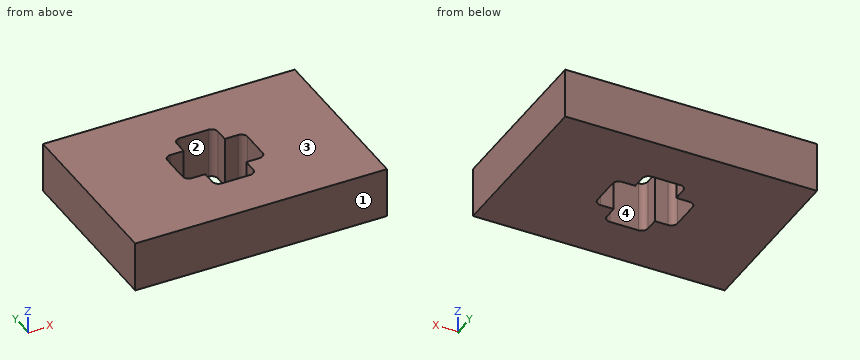
from build123d import *

# Parameters (mm, degrees)
SKETCH1_W           = 100
SKETCH1_H           = 70
BOSS_EXTRUDE1_DEPTH = 20


with BuildPart() as part:
    # Sketch1 → Boss-Extrude1 (new body)
    with BuildSketch(Plane.XY):
        Rectangle(SKETCH1_W, SKETCH1_H)
        with BuildLine():
            Line((-8.15, 13.4), (-8.15, 8.15))
            Line((-8.15, 8.15), (-13.4, 8.15))
            ThreePointArc((-13.4, 8.15), (-15.167766953, 7.417766953), (-15.9, 5.65))
            Line((-15.9, 5.65), (-15.9, -5.65))
            ThreePointArc((-15.9, -5.65), (-15.167766953, -7.417766953), (-13.4, -8.15))
            Line((-13.4, -8.15), (-8.15, -8.15))
            Line((-8.15, -8.15), (-8.15, -13.4))
            ThreePointArc((-8.15, -13.4), (-7.417766953, -15.167766953), (-5.65, -15.9))
            Line((-5.65, -15.9), (5.65, -15.9))
            ThreePointArc((5.65, -15.9), (7.417766953, -15.167766953), (8.15, -13.4))
            Line((8.15, -13.4), (8.15, -8.15))
            Line((8.15, -8.15), (13.4, -8.15))
            ThreePointArc((13.4, -8.15), (15.167766953, -7.417766953), (15.9, -5.65))
            Line((15.9, -5.65), (15.9, 5.65))
            ThreePointArc((15.9, 5.65), (15.167766953, 7.417766953), (13.4, 8.15))
            Line((13.4, 8.15), (8.15, 8.15))
            Line((8.15, 8.15), (8.15, 13.4))
            ThreePointArc((8.15, 13.4), (7.417766953, 15.167766953), (5.65, 15.9))
            Line((5.65, 15.9), (-5.65, 15.9))
            ThreePointArc((-5.65, 15.9), (-7.417766953, 15.167766953), (-8.15, 13.4))
        make_face(mode=Mode.SUBTRACT)
    extrude(amount=BOSS_EXTRUDE1_DEPTH)


solid = part.part
Verification items for the finished model (mm, model axes). Face numbers are marked on the shaded views. Give positions to 0.01 mm unless a question says otherwise; leave off trailing zeros. Loops run counter-clockwise (first coordinate to the right, second up) from the corner with the lowest first, then second, coordinate; pieces in that order, holes last.
1) Thickness scan on line 1 along Y through (x, z) = (-4.5, 6.5); line 2 along X through (y, z) = (2.5, 14.25); line 3 along X through (y, z) = (6.5, 3.5). Record the ranges inside material, lowest first.
2) Sectioned sample at B-B, the plane y = 0. Enter the section's corners in (x, z), then the cut area to 3 significant figures.
3) Sectioned sample at A-A, the plane z = 13. Enter the section's corners in (x, y).
4) Draft check along Y on the marked faces 1, 2, 3 and 4. Enter one of: pulls with the +Y half, pulls with the -Y half, needs draft (parallel to the pull), parting line crosses it, or undercut.
Answers:
1. line 1: y = -35 to -15.9, 15.9 to 35
1. line 2: x = -50 to -15.9, 15.9 to 50
1. line 3: x = -50 to -15.75, 15.75 to 50
2. outline: (-50, 0) - (-15.9, 0) - (-15.9, 20) - (-50, 20) - close; (15.9, 0) - (50, 0) - (50, 20) - (15.9, 20) - close
2. area: 1,360 mm2
3. outline: (-50, -35) - (50, -35) - (50, 35) - (-50, 35) - close; hole (-15.9, -5.65) arc R2.5 ccw to (-13.4, -8.15) - (-8.15, -8.15) - (-8.15, -13.4) arc R2.5 ccw to (-5.65, -15.9) - (5.65, -15.9) arc R2.5 ccw to (8.15, -13.4) - (8.15, -8.15) - (13.4, -8.15) arc R2.5 ccw to (15.9, -5.65) - (15.9, 5.65) arc R2.5 ccw to (13.4, 8.15) - (8.15, 8.15) - (8.15, 13.4) arc R2.5 ccw to (5.65, 15.9) - (-5.65, 15.9) arc R2.5 ccw to (-8.15, 13.4) - (-8.15, 8.15) - (-13.4, 8.15) arc R2.5 ccw to (-15.9, 5.65) - close
4. face 1: pulls with the -Y half
4. face 2: undercut
4. face 3: needs draft
4. face 4: undercut
